Build history of the part. All positions in model axes, mm. Round coordinates to 2 decimals unless told otherwise and drop trailing zeros. Write each loop counter-clockwise with the first axis right and the second up, starting at its lowest first coordinate (ties: lowest second). Pieces come first, ordered by that corner, then holes.
1) Saw through at C-C (y = 0.5). Write the cut outline in (x, z), plus the area to 3 significant figures.
2) Pull direction Z, two halves, no side cores. Call faces 1 (the cylindrical face through (0.86, 4.06, 38.99)), 2 (the flat face through (29, 8, 20)), 3 (the cylindrical face through (33.78, 4.06, 4.62)): +Z half, -Z half, draft (parallel to the pull), parting line (faces both ways), or undercut.
3) Saw through at B-B (x = 5). Write the cut outline in (y, z), plus the area to 3 significant figures.
4) Saw through at D-D (z = 23). Write the cut outline in (x, y).
5) Wall check: probe 1 along X at (y, z) = (6.75, 5); probe 2 along X at (y, z) = (7.5, 34); probe 3 along Z at (x, y) = (34, 7). Give the ranges that are in metal, low to high.
6) Saw through at A-A (x = 20). Write the cut outline in (y, z), plus the area to 3 significant figures.
from build123d import *

# Parameters (mm, degrees)
SKETCH1_W           = 40
SKETCH1_H           = 40
SKETCH1_R           = 8
BOSS_EXTRUDE1_DEPTH = 8
SKETCH12_R          = 1.25
CUT_EXTRUDE1_DEPTH  = 58.053472861
FILLET1_R           = 3


with BuildPart() as part:
    # Sketch1 → Boss-Extrude1 (new body)
    with BuildSketch(Plane(origin=(0, 0, 0), x_dir=(1, 0, 0), z_dir=(0, 1, 0))):
        with Locations((20, -19.888579387)):
            Rectangle(SKETCH1_W, SKETCH1_H)
        with Locations(Location((20, -19.888579387, 0), (0, 0, 270))):
            Circle(SKETCH1_R, mode=Mode.SUBTRACT)
    extrude(amount=BOSS_EXTRUDE1_DEPTH)

    # Sketch12 → Cut-Extrude1 (cut, through all)
    with BuildSketch(Plane(origin=(0, 8, 0), x_dir=(1, 0, 0), z_dir=(0, 1, 0))):
        with Locations(Location((5, -4.888579387, 0), (0, 0, 270))):
            Circle(SKETCH12_R)
        with Locations(Location((35, -4.888579387, 0), (0, 0, 270))):
            Circle(SKETCH12_R)
        with Locations(Location((35, -34.888579387, 0), (0, 0, 270))):
            Circle(SKETCH12_R)
        with Locations(Location((5, -34.888579387, 0), (0, 0, 270))):
            Circle(SKETCH12_R)
    extrude(amount=-CUT_EXTRUDE1_DEPTH, mode=Mode.SUBTRACT)

    # Fillet1
    fillet1_edges = [part.edges().sort_by_distance(p)[0] for p in [
        (0, 4, -0.111420613),
        (40, 4, -0.111420613),
        (40, 4, 39.888579387),
        (0, 4, 39.888579387),
    ]]
    fillet(fillet1_edges, radius=FILLET1_R)


solid = part.part
Evaluation:
1. outline: (0, 2.89) arc R3 ccw to (3, -0.11) - (37, -0.11) arc R3 ccw to (40, 2.89) - (40, 36.89) arc R3 ccw to (37, 39.89) - (3, 39.89) arc R3 ccw to (0, 36.89) - close; hole circle Ø2.5 at (5, 4.89); hole circle Ø2.5 at (5, 34.89); hole circle Ø16 at (20, 19.89); hole circle Ø2.5 at (35, 4.89); hole circle Ø2.5 at (35, 34.89)
1. area: 1,370 mm2
2. face 1: +Z half
2. face 2: draft
2. face 3: undercut
3. outline: (0, -0.11) - (8, -0.11) - (8, 3.64) - (0, 3.64) - close; (0, 6.14) - (8, 6.14) - (8, 33.64) - (0, 33.64) - close; (0, 36.14) - (8, 36.14) - (8, 39.89) - (0, 39.89) - close
3. area: 280 mm2
4. outline: (0, 0) - (12.63, 0) - (12.63, 8) - (0, 8) - close; (27.37, 0) - (40, 0) - (40, 8) - (27.37, 8) - close
5. probe 1: x = 0 to 3.75, 6.25 to 33.75, 36.25 to 40
5. probe 2: x = 0 to 4.12, 5.88 to 34.12, 35.88 to 40
5. probe 3: z = -0.11 to 4.14, 5.64 to 34.14, 35.64 to 39.89
6. outline: (0, -0.11) - (8, -0.11) - (8, 11.89) - (0, 11.89) - close; (0, 27.89) - (8, 27.89) - (8, 39.89) - (0, 39.89) - close
6. area: 192 mm2
